from build123d import *

# Parameters (mm, degrees)
CUT_EXTRUDE2_START = -20.2057
SKETCH2_R          = 2.7686
CUT_EXTRUDE2_DEPTH = 20.2057
FILLET1_R          = 2.3876
CHAMFER1_SIZE      = 0.762
CHAMFER2_SIZE      = 1.524


with BuildPart() as part:
    # Sketch1 → Revolve1 (revolve)
    with BuildSketch(Plane(origin=(0, 0, 0), x_dir=(0, 1, 0), z_dir=(0, 0, 1)), mode=Mode.PRIVATE) as revolve1_sk:
        Polygon((-25.0317, 0), (-25.0317, 8.7122), (-20.2057, 8.7122), (-20.2057, 24.6126), (-10.6807, 24.6126), (-10.6807, 12.7), (25.0317, 12.7), (25.0317, 0), align=None)
    revolve(revolve1_sk.sketch.rotate(Axis((0, -50.4317, 0), (0, 1, 0)), 270), axis=Axis((0, -50.4317, 0), (0, 1, 0)))

    # Sketch2 → Cut-Extrude2 (cut)
    with BuildSketch(Plane(origin=(0, 0, 0), x_dir=(-1, 0, 0), z_dir=(0, 1, 0)).offset(CUT_EXTRUDE2_START)):
        with Locations(Location((19.8374, 0, 0), (0, 0, 270))):
            Circle(SKETCH2_R)
        with Locations(Location((0, 19.8374, 0), (0, 0, 270))):
            Circle(SKETCH2_R)
        with Locations(Location((-19.8374, 0, 0), (0, 0, 270))):
            Circle(SKETCH2_R)
        with Locations(Location((0, -19.8374, 0), (0, 0, 270))):
            Circle(SKETCH2_R)
    extrude(amount=CUT_EXTRUDE2_DEPTH, mode=Mode.SUBTRACT)

    # Fillet1
    fillet1_edges = [part.edges().sort_by_distance(p)[0] for p in [
        (0, -10.6807, 12.7),
    ]]
    fillet(fillet1_edges, radius=FILLET1_R)

    # Chamfer1
    chamfer1_edges = [part.edges().sort_by_distance(p)[0] for p in [
        (0, -10.6807, 24.6126),
        (0, -20.2057, 24.6126),
    ]]
    chamfer(chamfer1_edges, length=CHAMFER1_SIZE)

    # Chamfer2
    chamfer2_edges = [part.edges().sort_by_distance(p)[0] for p in [
        (0, 25.0317, 12.7),
    ]]
    chamfer(chamfer2_edges, length=CHAMFER2_SIZE)


solid = part.part
The model under review builds one solid part; all positions refer to its coordinate system, in mm. A direction names the side the tool comes from. Round coordinates to 2 decimals unless told otherwise and drop trailing zeros. Write each loop counter-clockwise with the first axis right and the second up, starting at its lowest first coordinate (ties: lowest second). Pieces come first, ordered by that corner, then holes. Notation, with made-up numbers: (-23, 62.25) - (23, 62.25) arc R28 cw to (23, 89.25) - close; hole circle Ø3 at (72, 47). An arc over 180 degrees is marked (long way). One line per item, written item: value. Start each with the question number.
1. Machinability: for faces 1 (the face through (-2.62, -22.58, -8.31)), 2 (the face through (7.7, 7.8, 10.1)), 3 (the face through (0, -25.032, 0)), which of the approach directions +Z, -Z, +X, -X, +Y, -Y give a long, thin tool a straight path to every point of the face, cutting with its end or side? Answer none if there is none.
2. The part is to be moulded in two halves that separate along X. For faces 4 (the face through (-16.634, -15.387, 18.141)), 5 (the face through (0, -20.206, 10)), 6 (the face through (17.503, -15.51, -1.488)), 7 (the face through (-0.832, -15.51, 17.197)), say which applies: released by +X, released by -X, zero draft, split by the parting line, or undercut.
3. Clearance check with flat-ended pins moving along their axes: P1, Ø3.5, axis at x = 0, z = 19.84, coming from the +Y side; P2, Ø10, axis at y = -19, z = -17, coming from the -X side; P3, Ø12, axis at x = 9, y = -1.5, coming from the -Z side; P4, Ø3, axis at y = 4, z = -7, coming from the -X side. State where each tip first meets the part, or that it passes through.
4. Consider section A-A on x = 0. Write out the cut boundary in (y, z).
5. Consider section C-C on y = 22.5. Write out the cut boundary in (x, z).
6. Consider section B-B on z = 0. Write out the cut boundary in (x, y).
7. To check wall thickness, follow L1, parallel to X at y = -12.75, z = 0; L2, parallel to Y at x = 9, z = 0; L3, parallel to X at y = 5, z = 6. State the ranges of each line that lie inside material, in increasing order. Write a range as from..to.
Checks:
1. face 1: -Y
1. face 2: +Y
1. face 3: +Z, -Z, +X, -X, -Y
2. face 4: split by the parting line
2. face 5: zero draft
2. face 6: undercut
2. face 7: undercut
3. P1: passes through
3. P2: stops at x = -21.49
3. P3: stops at z = -12.34
3. P4: stops at x = -11.45
4. outline: (-25.03, -8.71) - (-20.21, -8.71) - (-20.21, -17.07) - (-10.68, -17.07) - (-10.68, -15.09) arc R2.39 cw to (-8.29, -12.7) - (23.51, -12.7) - (25.03, -11.18) - (25.03, 11.18) - (23.51, 12.7) - (-8.29, 12.7) arc R2.39 cw to (-10.68, 15.09) - (-10.68, 17.07) - (-20.21, 17.07) - (-20.21, 8.71) - (-25.03, 8.71) - close; (-20.21, -23.85) - (-19.44, -24.61) - (-11.44, -24.61) - (-10.68, -23.85) - (-10.68, -22.61) - (-20.21, -22.61) - close; (-20.21, 22.61) - (-10.68, 22.61) - (-10.68, 23.85) - (-11.44, 24.61) - (-19.44, 24.61) - (-20.21, 23.85) - close
5. outline: circle Ø25.4 at (0, 0)
6. outline: (-24.61, -19.44) - (-23.85, -20.21) - (-22.61, -20.21) - (-22.61, -10.68) - (-23.85, -10.68) - (-24.61, -11.44) - close; (-17.07, -20.21) - (-8.71, -20.21) - (-8.71, -25.03) - (8.71, -25.03) - (8.71, -20.21) - (17.07, -20.21) - (17.07, -10.68) - (15.09, -10.68) arc R2.39 cw to (12.7, -8.29) - (12.7, 23.51) - (11.18, 25.03) - (-11.18, 25.03) - (-12.7, 23.51) - (-12.7, -8.29) arc R2.39 cw to (-15.09, -10.68) - (-17.07, -10.68) - close; (22.61, -20.21) - (23.85, -20.21) - (24.61, -19.44) - (24.61, -11.44) - (23.85, -10.68) - (22.61, -10.68) - close
7. L1: x = -24.61..-22.61, -17.07..17.07, 22.61..24.61
7. L2: y = -20.21..25.03
7. L3: x = -11.19..11.19
